Autodesk Inventor part; units mm, degrees
ref_plane "YZ Plane" through (0, 0, 0) normal (1, 0, 0) x (0, 1, 0)
ref_plane "XZ Plane" through (0, 0, 0) normal (0, 1, 0) x (-1, 0, 0)
ref_plane "XY Plane" through (0, 0, 0) normal (0, 0, 1) x (1, 0, 0)
sketch "Sketch1" plane through (0, 0, 0) normal (0, 1, 0) x (-1, 0, 0)
  line L0 (6.35, -451.5) -> (-6.35, -451.5)
  line L1 (-6.35, -451.5) -> (-6.35, 451.5)
  line L2 (-6.35, 451.5) -> (6.35, 451.5)
  line L3 (6.35, 451.5) -> (6.35, -451.5)
  line L4 (6.35, -451.5) -> (-6.35, 451.5) construction
  line L5 (-6.35, -451.5) -> (6.35, 451.5) construction
  point P0 (0, 0)
  dimension "d0" = 12.7
  dimension "d1" = 903
extrude "Extrusion1" add sketch "Sketch1" along normal blind 12.7
sketch "Sketch2" plane through (0, 12.7, 0) normal (0, 1, 0) x (1, 0, 0)
  circle A0 centre (0, -434.99) radius 2.5
  line L0 (-6.35, -451.5) -> (6.35, -451.5)
  point P0 (0, 0)
  dimension "d4" = 5
  dimension "d5" = 16.51
sketch "Sketch3" plane through (0, 12.7, 0) normal (0, 1, 0) x (1, 0, 0)
  circle A0 centre (0, -396.89) radius 2.5
  line L0 (-6.35, -451.5) -> (6.35, -451.5)
  point P0 (0, 0)
  dimension "d6" = 5
  dimension "d7" = 54.61
sketch "Sketch4" plane through (0, 12.7, 0) normal (0, 1, 0) x (1, 0, 0)
  circle A0 centre (0, -320.84) radius 2.5
  line L0 (-6.35, -451.5) -> (6.35, -451.5)
  point P0 (0, 0)
  dimension "d8" = 5
  dimension "d9" = 130.66
sketch "Sketch5" plane through (0, 12.7, 0) normal (0, 1, 0) x (1, 0, 0)
  circle A0 centre (0, -193.84) radius 2.5
  line L0 (-6.35, -451.5) -> (6.35, -451.5)
  point P0 (0, 0)
  dimension "d10" = 5
  dimension "d11" = 257.66
sketch "Sketch6" plane through (0, 12.7, 0) normal (0, 1, 0) x (1, 0, 0)
  circle A0 centre (0, -66.84) radius 2.5
  line L0 (-6.35, -451.5) -> (6.35, -451.5)
  point P0 (0, 0)
  dimension "d12" = 5
  dimension "d13" = 384.66
sketch "Sketch7" plane through (0, 12.7, 0) normal (0, 1, 0) x (1, 0, 0)
  circle A0 centre (0, 60.16) radius 2.5
  line L0 (-6.35, -451.5) -> (6.35, -451.5)
  point P0 (0, 0)
  dimension "d14" = 5
  dimension "d15" = 511.66
sketch "Sketch8" plane through (0, 12.7, 0) normal (0, 1, 0) x (1, 0, 0)
  circle A0 centre (0, 187.16) radius 2.5
  line L0 (-6.35, -451.5) -> (6.35, -451.5)
  point P0 (0, 0)
  dimension "d16" = 5
  dimension "d17" = 638.66
sketch "Sketch9" plane through (0, 12.7, 0) normal (0, 1, 0) x (1, 0, 0)
  circle A0 centre (0, 205.24) radius 2.5
  line L0 (-6.35, -451.5) -> (6.35, -451.5)
  point P0 (0, 0)
  dimension "d18" = 5
  dimension "d19" = 656.74
sketch "Sketch10" plane through (0, 12.7, 0) normal (0, 1, 0) x (1, 0, 0)
  circle A0 centre (0, 230.64) radius 2.5
  line L0 (-6.35, -451.5) -> (6.35, -451.5)
  point P0 (0, 0)
  dimension "d20" = 5
  dimension "d21" = 682.14
hole "Hole1" at (0, 12.7, 434.99) direction (0, -1, 0) diameter 5 end through all
hole "Hole2" at (0, 12.7, 396.89) direction (0, -1, 0) diameter 5 end through all
hole "Hole3" at (0, 12.7, 320.84) direction (0, -1, 0) diameter 5 end through all
hole "Hole4" at (0, 12.7, 193.84) direction (0, -1, 0) diameter 5 end through all
hole "Hole5" at (0, 12.7, 66.84) direction (0, -1, 0) diameter 5 end through all
hole "Hole6" at (0, 12.7, -60.16) direction (0, -1, 0) diameter 5 end through all
hole "Hole7" at (0, 12.7, -187.16) direction (0, -1, 0) diameter 5 end through all
hole "Hole8" at (0, 12.7, -205.24) direction (0, -1, 0) diameter 5 end through all
hole "Hole9" at (0, 12.7, -230.64) direction (0, -1, 0) diameter 5 end through all
sketch "Sketch11" plane through (6.35, 0, -451.5) normal (0, 0, -1) x (-1, 0, 0)
  circle A0 centre (6.35, 6.35) radius 1.5
  line L0 (0, 0) -> (0, 12.7)
  point P0 (6.35, 0)
  dimension "d85" = 3
  dimension "d86" = 6.35
  dimension "d87" = 6.35
hole "Hole10" at (0, 6.35, -451.5) direction (0, 0, 1) diameter 3 depth 8 tip angle 118
thread "Thread1"
sketch "Sketch12" plane through (6.35, 0, 451.5) normal (1, 0, 0) x (0, 0, -1)
  circle A0 centre (194.16, 7.3065) radius 2.5
  line L0 (0, 0) -> (0, 12.7)
  point P0 (451.5, 0)
  dimension "d97" = 5
  dimension "d98" = 194.16
sketch "Sketch13" plane through (6.35, 0, 451.5) normal (1, 0, 0) x (0, 0, -1)
  circle A0 centre (321.16, 7.3065) radius 2.5
  line L0 (0, 0) -> (0, 12.7)
  point P0 (451.5, 0)
  dimension "d99" = 5
  dimension "d100" = 321.16
sketch "Sketch14" plane through (6.35, 0, 451.5) normal (1, 0, 0) x (0, 0, -1)
  circle A0 centre (448.16, 7.3065) radius 2.5
  line L0 (0, 0) -> (0, 12.7)
  point P0 (451.5, 0)
  dimension "d101" = 5
  dimension "d102" = 448.16
sketch "Sketch15" plane through (6.35, 0, 451.5) normal (1, 0, 0) x (0, 0, -1)
  circle A0 centre (575.16, 7.3065) radius 2.5
  line L0 (0, 0) -> (0, 12.7)
  point P0 (451.5, 0)
  dimension "d103" = 5
  dimension "d104" = 575.16
hole "Hole11" at (6.35, 7.3065, 257.34) direction (-1, 0, 0) diameter 5 end through all
hole "Hole12" at (6.35, 7.3065, 130.34) direction (-1, 0, 0) diameter 5 end through all
hole "Hole13" at (6.35, 7.3065, 3.34) direction (-1, 0, 0) diameter 5 end through all
hole "Hole14" at (6.35, 7.3065, -123.66) direction (-1, 0, 0) diameter 5 end through all
properties part number "Plate Support"
Input: part model. Units: mm. Frame: model coordinates. Coordinates: 2 decimals unless noted, no trailing zeros.
1. Cut plane A-A, the plane y = 2. Count the separate pieces of the cut face and the enclosed holes in it, plus the area to 3 significant figures.
Checked values:
separate pieces: 1
enclosed holes: 9
area: 11,300 mm2
2. Contact query for flat-ended pins moving along their axis: P1, Ø4.5, axis at x = 0, z = -187.16, coming from the +Y side; P2, Ø2, axis at x = 1, y = 6, coming from the -Z side; P3, Ø1.8, axis at x = 0, y = 6.35, coming from the -Z side. Output: stop coordinate, or through.
Checked values:
P1: passes through
P2: stops at z = -451.5
P3: stops at z = -443.14
3. Ray query, line 1 along Z through (x, y) = (3.25, 6.75); line 2 along Z through (x, y) = (-5.5, 8); line 3 along X through (y, z) = (10.25, 396.89). Return the intervals inside material, ascending.
Checked values:
line 1: z = -451.5 to -126.1, -121.22 to 0.9, 5.78 to 127.9, 132.78 to 254.9, 259.78 to 451.5
line 2: z = -451.5 to -126.06, -121.26 to 0.94, 5.74 to 127.94, 132.74 to 254.94, 259.74 to 451.5
line 3: x = -6.35 to -2.5, 2.5 to 6.35
